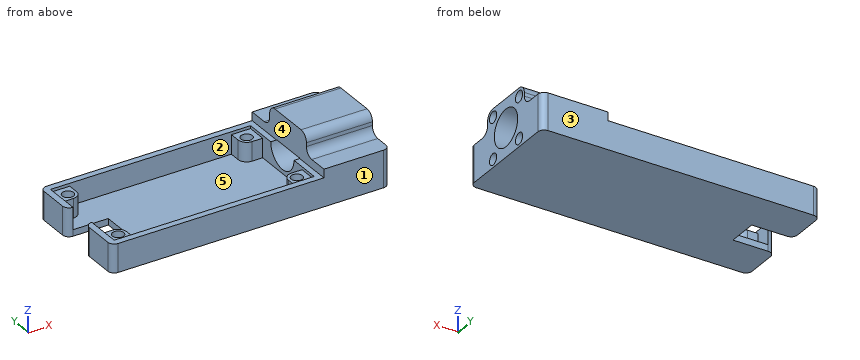
```python
from build123d import *

# Parameters (mm, degrees)
BODY_DEPTH          = 10
PCB_RECESS_DEPTH    = 7.75
SKETCH11_R          = 3.000000000000004
SKETCH11_R_2        = 2.999999999999999
SKETCH11_R_3        = 3.000000000000008
SKETCH11_R_4        = 3.0000000000000084
PCB_BOSS_DEPTH      = 6.75
FILLET2_R           = 2.25
BOSS_EXTRUDE2_DEPTH = 23.25
BOSS_EXTRUDE3_DEPTH = 3
SKETCH25_R          = 6.5
CUT_EXTRUDE9_DEPTH  = 15
CUT_EXTRUDE10_DEPTH = 10.25
FILLET7_R           = 3
FILLET8_R           = 2.25
SKETCH27_R          = 2.0000000000000067
SKETCH27_R_2        = 2.000000000000003
SKETCH27_R_3        = 2
SKETCH27_R_4        = 1.9999999999999996
CUT_EXTRUDE11_DEPTH = 5.5
SKETCH12_R          = 1.9999999999999991
SKETCH12_R_2        = 1.9999999999999967
SKETCH12_R_3        = 1.9999999999999996
CUT_EXTRUDE5_DEPTH  = 4.5


with BuildPart() as part:
    # Sketch4 → body (new body)
    with BuildSketch(Plane.XY):
        Polygon((0, 40), (1.73e-15, 25.25), (14.7, 25.25), (14.7, 14.750000000000002), (0, 14.75), (0, 0), (97.99999999999999, 6.94e-15), (98, 40.00000000000001), align=None)
    extrude(amount=BODY_DEPTH)

    # Sketch10 → pcb-recess (cut)
    with BuildSketch(Plane.XY.offset(10)):
        Polygon((72.75000000000001, 2.250000000000009), (2.2500000000000018, 2.2500000000000004), (2.2500000000000044, 37.74999999999999), (72.75, 37.75000000000001), align=None)
    extrude(amount=-PCB_RECESS_DEPTH, mode=Mode.SUBTRACT)

    # Sketch11 → pcb-boss (add)
    with BuildSketch(Plane.XY.offset(2.25)):
        with Locations((6.000000000000004, 34)):
            Circle(SKETCH11_R)
        with BuildLine():
            Line((2.250000000000004, 31), (6.000000000000004, 31))
            ThreePointArc((6.0000000000000036, 30.999999999999996), (3.8786796564403594, 36.121320343559645), (9.000000000000009, 34))
            Line((9.000000000000007, 34), (9.000000000000007, 37.74999999999999))
            Line((9.000000000000007, 37.74999999999999), (2.2500000000000044, 37.74999999999999))
            Line((2.2500000000000044, 37.74999999999999), (2.250000000000004, 31))
        make_face()
        with BuildLine():
            Line((2.2500000000000018, 2.2500000000000004), (9.000000000000007, 2.2500000000000013))
            Line((9.000000000000007, 2.2500000000000013), (9.000000000000007, 6.000000000000005))
            ThreePointArc((9.000000000000007, 6.000000000000004), (3.8786796564403647, 3.8786796564403634), (6.000000000000007, 9.000000000000004))
            Line((6.000000000000007, 9.000000000000005), (2.250000000000002, 9.000000000000014))
            Line((2.250000000000002, 9.000000000000014), (2.2500000000000018, 2.25))
        make_face()
        with Locations((6.000000000000007, 6.000000000000005)):
            Circle(SKETCH11_R_2)
        with Locations((69, 6.000000000000005)):
            Circle(SKETCH11_R_3)
        with BuildLine():
            Line((72.75000000000001, 2.250000000000009), (72.75000000000001, 9.000000000000012))
            Line((72.75000000000001, 9.000000000000012), (69, 9.000000000000012))
            ThreePointArc((69, 9.000000000000014), (71.12132034355965, 8.121320343559653), (72.00000000000001, 6.000000000000005))
            ThreePointArc((72.00000000000001, 6.000000000000004), (69, 2.9999999999999973), (65.99999999999999, 6.000000000000005))
            Line((66, 6.000000000000005), (66, 2.250000000000008))
            Line((66, 2.250000000000008), (72.75000000000001, 2.250000000000009))
        make_face()
        with BuildLine():
            Line((72.75, 37.75000000000001), (66, 37.75000000000001))
            Line((66, 37.75000000000001), (66, 34))
            ThreePointArc((65.99999999999999, 34), (69, 37.00000000000001), (72.00000000000001, 34))
            ThreePointArc((72.00000000000001, 34), (71.12132034355965, 31.87867965644035), (69, 30.999999999999993))
            Line((69, 30.999999999999993), (72.75, 30.999999999999993))
            Line((72.75, 30.999999999999993), (72.75, 37.75000000000001))
        make_face()
        with Locations((69, 34)):
            Circle(SKETCH11_R_4)
    extrude(amount=PCB_BOSS_DEPTH)

    # Fillet2
    fillet2_edges = [part.edges().sort_by_distance(p)[0] for p in [
        (0, 14.75, 5),
        (1.73e-15, 25.25, 5),
    ]]
    fillet(fillet2_edges, radius=FILLET2_R - 0.0001)  # a hair under: the kernel refuses the full size

    # Sketch23 → Boss-Extrude2 (add)
    with BuildSketch(Plane(origin=(97.99999999999999, -3.4e-14, 0), x_dir=(0, 0, -1), z_dir=(1, -3.5e-16, 0))):
        Polygon((-10, 30.250000000000025), (-20.299999999999997, 30.25000000000003), (-20.299999999999994, 9.750000000000027), (-9.999999999999998, 9.75000000000002), align=None)
    extrude(amount=-BOSS_EXTRUDE2_DEPTH)

    # Sketch24 → Boss-Extrude3 (add)
    with BuildSketch(Plane.XY.offset(10)):
        Polygon((74.75, 30.25), (98, 30.25), (98, 40.00000000000001), (74.75, 39.99999999999999), align=None)
        Polygon((74.75000000000001, 9.749999999999995), (97.99999999999999, 9.749999999999995), (97.99999999999999, 6.94e-15), (74.75000000000001, -6.94e-15), align=None)
    extrude(amount=BOSS_EXTRUDE3_DEPTH)

    # Sketch25 → Cut-Extrude9 (cut)
    with BuildSketch(Plane(origin=(97.99999999999999, -3.4e-14, 0), x_dir=(0, 0, -1), z_dir=(1, -3.5e-16, 0))):
        with Locations(Location((-10.149999999999999, 20.000000000000025, 0), (0, 0, 90))):
            Circle(SKETCH25_R)
    extrude(amount=-CUT_EXTRUDE9_DEPTH, mode=Mode.SUBTRACT)

    # Sketch26 → Cut-Extrude10 (cut)
    with BuildSketch(Plane(origin=(83, -2.88e-14, 0), x_dir=(0, 0, -1), z_dir=(1, -3.5e-16, 0))):
        with BuildLine():
            Line((-10.149999999999999, 26.500000000000025), (-10.149999999999999, 13.500000000000027))
            ThreePointArc((-10.149999999999999, 13.500000000000027), (-3.6499999999999986, 20.000000000000025), (-10.149999999999999, 26.500000000000025))
        make_face()
    extrude(amount=-CUT_EXTRUDE10_DEPTH, mode=Mode.SUBTRACT)

    # Fillet7
    fillet7_edges = [part.edges().sort_by_distance(p)[0] for p in [
        (86.37499999999999, 9.749999999999996, 20.299999999999994),
        (86.375, 30.249999999999996, 20.299999999999997),
        (86.375, 30.25, 13),
        (86.375, 9.749999999999995, 13),
    ]]
    fillet(fillet7_edges, radius=FILLET7_R)

    # Fillet8
    fillet8_edges = [part.edges().sort_by_distance(p)[0] for p in [
        (0, 40, 5),
        (98, 40.00000000000001, 6.5),
        (97.99999999999999, 6.94e-15, 6.5),
        (0, 0, 5),
    ]]
    fillet(fillet8_edges, radius=FILLET8_R)

    # Sketch27 → Cut-Extrude11 (cut)
    with BuildSketch(Plane(origin=(97.99999999999999, -3.4e-14, 0), x_dir=(0, 0, -1), z_dir=(1, -3.5e-16, 0))):
        with Locations(Location((-17.350000000000005, 27.300000000000026, 0), (0, 0, 90))):
            Circle(SKETCH27_R)
        with Locations(Location((-2.850000000000002, 27.300000000000026, 0), (0, 0, 90))):
            Circle(SKETCH27_R_2)
        with Locations(Location((-2.8499999999999948, 12.800000000000026, 0), (0, 0, 90))):
            Circle(SKETCH27_R_3)
        with Locations(Location((-17.349999999999998, 12.800000000000026, 0), (0, 0, 90))):
            Circle(SKETCH27_R_4)
    extrude(amount=-CUT_EXTRUDE11_DEPTH, mode=Mode.SUBTRACT)

    # Sketch12 → Cut-Extrude5 (cut)
    with BuildSketch(Plane.XY.offset(9.000000000000002)):
        with Locations((6.000000000000004, 34)):
            Circle(SKETCH12_R)
        with Locations((69, 34)):
            Circle(SKETCH12_R_2)
        with Locations((69, 6.000000000000005)):
            Circle(SKETCH12_R_2)
        with Locations((6.000000000000007, 6.000000000000005)):
            Circle(SKETCH12_R_3)
    extrude(amount=-CUT_EXTRUDE5_DEPTH, mode=Mode.SUBTRACT)


solid = part.part
```
Geometry check sheet. Reference: the model listing, model coordinates, mm. Face numbers are marked on the shaded views. A direction names the side the tool comes from. Coordinates: 2 decimals unless noted, no trailing zeros. Order: outer loops, then holes, each group sorted by start corner. A loop starts at its lowest first (then second) coordinate and runs counter-clockwise, first axis right, second up. Notation, with made-up numbers: (31, -22) - (83, -22) arc R24 ccw to (83, -6) - close; hole circle Ø11 at (-10, -3). An arc over 180 degrees is marked (long way). Answer in a Markdown table with one row per item. Add a question column.
1. Section check A-A (x = 28). Enter the section's corners in (y, z), plus the area to 3 significant figures.
2. Draft check along Y on the marked faces 3, 4 and 5. Enter one of: +Y half, -Y half, draft (parallel to the pull), parting line (faces both ways), or undercut.
3. Access from +Z, -Z, +X, -X, +Y, -Y to the whole of each face (thin tool, end or side, straight path). Record for the marked faces 1 and 2.
4. Section check B-B (y = 20). Enter the section's corners in (x, z).
5. Material ranges on L1, parallel to Z at x = 95.3, y = 27.3; L2, parallel to X at y = 9.5, z = 5.5; L3, parallel to Z at x = 31.5, y = 17, recorded low to high. Write a range as [from, to].
6. Gauge pin test, flat ends, axial feed: pin 1 Ø3 at (y, z) = (27.3, 2.85) entering from +X; pin 2 Ø3.5 at (x, y) = (6, 6) entering from +Z; pin 3 Ø4 at (x, y) = (79, 21) entering from -Z; pin 4 Ø3.5 at (x, y) = (68, 33) entering from +Z. Record the tip position at first contact, or that the pin passes through.
Data:
| question | item | result |
|---|---|---|
| 1 | outline | (0, 0) - (40, 0) - (40, 10) - (37.75, 10) - (37.75, 2.25) - (2.25, 2.25) - (2.25, 10) - (0, 10) - close |
| 1 | area | 125 mm² |
| 2 | face 3 | +Y half |
| 2 | face 4 | draft |
| 2 | face 5 | undercut |
| 3 | face 1 | +Z, -Z, +X, -X, -Y |
| 3 | face 2 | +Z |
| 4 | outline | (14.7, 0) - (98, 0) - (98, 3.65) - (72.75, 3.65) - (72.75, 2.25) - (14.7, 2.25) - close; (74.75, 10.15) - (83, 10.15) - (83, 16.65) - (98, 16.65) - (98, 20.3) - (74.75, 20.3) - close |
| 5 | L1 | z = [0, 0.85], [4.85, 15.35], [19.35, 20.3] |
| 5 | L2 | x = [0, 2.25], [72.75, 98] |
| 5 | L3 | z = [0, 2.25] |
| 6 | pin 1 | stops at x = 92.5 |
| 6 | pin 2 | stops at z = 4.5 |
| 6 | pin 3 | stops at z = 0 |
| 6 | pin 4 | stops at z = 9 |
